The listing builds one solid part. Answer for the finished solid, in the listing's coordinates (mm). Face numbers are marked on the shaded views. A direction names the side the tool comes from. Give positions to 0.01 mm unless a question says otherwise; leave off trailing zeros. Order: outer loops, then holes, each group sorted by start corner. A loop starts at its lowest first (then second) coordinate and runs counter-clockwise, first axis right, second up. Notation, with made-up numbers: (76, -14) - (94, -14) arc R8 cw to (94, -1) - close; hole circle Ø3 at (75, 76.5). An arc over 180 degrees is marked (long way). Use a Markdown table: item, result. Add a question column.
1) The mould has two halves that part along X. Classify the marked faces 3, 4, 5 and 6: released by +X, released by -X, zero draft, split by the parting line, or undercut.
2) Flat-ended cylindrical pins translate along their axes: pin 1 (9.5 mm diameter, centred on x = -63.5, z = 14.5, fed in from +Y); pin 2 (2.5 mm diameter, centred on x = 52.48, z = 9.52, fed in from +Y); pin 3 (3 mm diameter, centred on x = 47.5, z = 13.5, fed in from +Y). Find the tip coordinate at first contact, or state that the pin passes through.
3) For the marked faces 1 and 2, determine the directions among +Z, -Z, +X, -X, +Y, -Y from which every point of the face is accessible in a straight line to the end or side of a thin tool.
4) Find section A-A, the plane z = 4. State how many separate pieces and enclosed holes the cut face has, plus the area to 3 significant figures.
5) Find section D-D, the plane x = 109. Determine the outline of the cut face in (y, z), plus the area to 3 significant figures.
6) Straight lines are drawn through the part: line 1 (Y direction, x = 57, z = 5); line 2 (Y direction, x = 0, z = 6.5); line 3 (Y direction, x = -122, z = 9.25). For each, find the intervals that lie inside material, in ascending order.
7) Find section C-C, the plane x = 59.5. Determine the outline of the cut face in (y, z), plus the area to 3 significant figures.
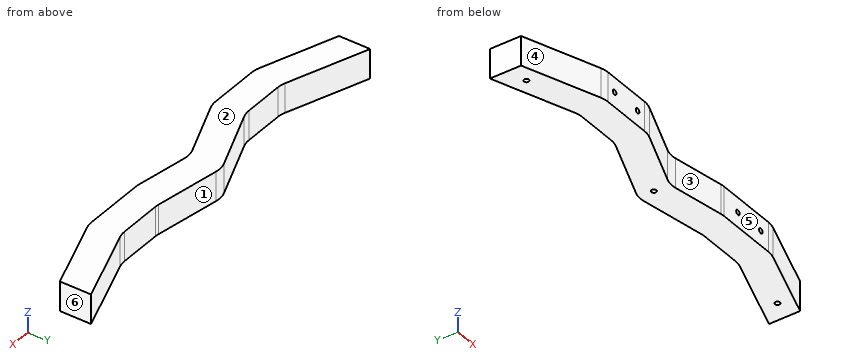
from build123d import *

# Parameters (mm, degrees)
BOSS_EXTRUDE1_DEPTH              = 19.05
F_1_8_0_125_DIAMETER_HOLE1_D     = 3.175
F_1_8_0_125_DIAMETER_HOLE1_DEPTH = 11.1252
F_1_8_0_125_DIAMETER_HOLE1_TIP   = 0.953866233
FILLET1_R                        = 15.875
F_1_8_0_125_DIAMETER_HOLE2_D     = 3.175
F_1_8_0_125_DIAMETER_HOLE2_DEPTH = 11.1252
F_1_8_0_125_DIAMETER_HOLE2_TIP   = 0.953866233
F_1_8_0_125_DIAMETER_HOLE3_D     = 3.175
F_1_8_0_125_DIAMETER_HOLE3_DEPTH = 11.1252
F_1_8_0_125_DIAMETER_HOLE3_TIP   = 0.953866233


with BuildPart() as part:
    # Sketch1 → Boss-Extrude1 (new body)
    with BuildSketch(Plane.XY):
        Polygon((0, 0), (47.625, -7.9375), (79.375, -7.9375), (133.35, 11.1125), (133.35, -9.089191705), (82.638126498, -26.9875), (38.820132509, -26.9875), (0, -20.517477915), (-43.956305212, -38.1), (-82.638126498, -38.1), (-133.35, -20.201691705), (-133.35, 0), (-79.375, -19.05), (-47.625, -19.05), align=None)
    extrude(amount=BOSS_EXTRUDE1_DEPTH)

    # 1/8 (0.125) Diameter Hole1
    with Locations(Plane(origin=(0, 0, 0), x_dir=(-1, 0, 0), z_dir=(0, 0, -1))):
        with Locations((-120.65, -3.470698794), (0, -10.258738958), (120.65, -14.583198794)):
            Hole(F_1_8_0_125_DIAMETER_HOLE1_D / 2, depth=F_1_8_0_125_DIAMETER_HOLE1_DEPTH)
            with Locations((0, 0, -(F_1_8_0_125_DIAMETER_HOLE1_DEPTH + F_1_8_0_125_DIAMETER_HOLE1_TIP / 2))):  # 118° drill point
                Cone(0, F_1_8_0_125_DIAMETER_HOLE1_D / 2, F_1_8_0_125_DIAMETER_HOLE1_TIP, mode=Mode.SUBTRACT)

    # Fillet1
    fillet1_edges = [part.edges().sort_by_distance(p)[0] for p in [
        (0, 0, 9.525),
        (47.625, -7.9375, 9.525),
        (79.375, -7.9375, 9.525),
        (82.638126498, -26.9875, 9.525),
        (38.820132509, -26.9875, 9.525),
        (0, -20.517477915, 9.525),
        (-43.956305212, -38.1, 9.525),
        (-82.638126498, -38.1, 9.525),
        (-79.375, -19.05, 9.525),
        (-47.625, -19.05, 9.525),
    ]]
    fillet(fillet1_edges, radius=FILLET1_R)

    # 1/8 (0.125) Diameter Hole2
    with Locations(Plane(origin=(0, -26.9875, 0), x_dir=(-1, 0, 0), z_dir=(0, -1, 0))):
        with Locations((-73.116041543, -9.525), (-52.478541543, -9.525)):
            Hole(F_1_8_0_125_DIAMETER_HOLE2_D / 2, depth=F_1_8_0_125_DIAMETER_HOLE2_DEPTH)
            with Locations((0, 0, -(F_1_8_0_125_DIAMETER_HOLE2_DEPTH + F_1_8_0_125_DIAMETER_HOLE2_TIP / 2))):  # 118° drill point
                Cone(0, F_1_8_0_125_DIAMETER_HOLE2_D / 2, F_1_8_0_125_DIAMETER_HOLE2_TIP, mode=Mode.SUBTRACT)

    # 1/8 (0.125) Diameter Hole3
    with Locations(Plane(origin=(0, -38.1, 0), x_dir=(-1, 0, 0), z_dir=(0, -1, 0))):
        with Locations((53.350236787, -9.525), (73.987736787, -9.525)):
            Hole(F_1_8_0_125_DIAMETER_HOLE3_D / 2, depth=F_1_8_0_125_DIAMETER_HOLE3_DEPTH)
            with Locations((0, 0, -(F_1_8_0_125_DIAMETER_HOLE3_DEPTH + F_1_8_0_125_DIAMETER_HOLE3_TIP / 2))):  # 118° drill point
                Cone(0, F_1_8_0_125_DIAMETER_HOLE3_D / 2, F_1_8_0_125_DIAMETER_HOLE3_TIP, mode=Mode.SUBTRACT)


solid = part.part
The answers:
| question | item | result |
|---|---|---|
| 1 | face 3 | undercut |
| 1 | face 4 | released by -X |
| 1 | face 5 | zero draft |
| 1 | face 6 | released by +X |
| 2 | pin 1 | y = -19.05 |
| 2 | pin 2 | y = -7.94 |
| 2 | pin 3 | y = -7.67 |
| 3 | face 1 | +Z, -Z, +Y |
| 3 | face 2 | +Z, +X, -X, +Y, -Y |
| 4 | separate pieces | 1 |
| 4 | enclosed holes | 3 |
| 4 | area | 5,310 mm2 |
| 5 | outline | (-17.68, 0) - (2.52, 0) - (2.52, 19.05) - (-17.68, 19.05) - close |
| 5 | area | 385 mm2 |
| 6 | line 1 | -26.99 to -7.94 |
| 6 | line 2 | -21.13 to -11.85, -8.67 to -0.61 |
| 6 | line 3 | -24.21 to -15.42, -13.75 to -4.01 |
| 7 | outline | (-26.99, 0) - (-7.94, 0) - (-7.94, 19.05) - (-26.99, 19.05) - close |
| 7 | area | 363 mm2 |
